```python
from build123d import *

# Parameters (mm, degrees)
SALIENTE_EXTRUIR1_DEPTH    = 3
SALIENTE_EXTRUIR2_DEPTH    = 3
NERVIO6_START              = -1.25
NERVIO6_DEPTH              = 2.5
NERVIO7_START              = -2
NERVIO7_DEPTH              = 4
CROQUIS3_R                 = 1.5875
CORTAR_EXTRUIR1_DEPTH      = 12
CORTAR_EXTRUIR2_DEPTH      = 10
CORTAR_EXTRUIR2_DEPTH_BACK = 12


# Read off the part's stored shape, not the designer's step: Nervio6, Nervio7
with BuildPart() as part:
    # Croquis1 → Saliente-Extruir1 (new body)
    with BuildSketch(Plane.XY):
        Polygon((-20, 5), (-20, -5), (20, -5), (20, 5), (0, 5), align=None)
        Polygon((-15, 30), (-20, 5), (0, 5), (0, 30), align=None)
        Polygon((0, 5), (20, 5), (15, 30), (0, 30), align=None)
    extrude(amount=SALIENTE_EXTRUIR1_DEPTH)

    # Croquis2 → Saliente-Extruir2 (add)
    with BuildSketch(Plane.XY.offset(3)):
        Polygon((-19.6, 7), (-20, 5), (20, 5), (19.6, 7), align=None)
    extrude(amount=SALIENTE_EXTRUIR2_DEPTH)

    # Nervio6 outline → Nervio6 (add)
    with BuildSketch(Plane(origin=(16, 0, 0), x_dir=(0, 0, -1), z_dir=(1, 0, 0)).offset(NERVIO6_START)):
        with BuildLine():
            Line((-3, 7), (-3, 18.5))
            ThreePointArc((-3, 18.5), (-3.776888017, 12.561362091), (-6, 7))
            Line((-6, 7), (-3, 7))
        make_face()
    nervio6 = extrude(amount=NERVIO6_DEPTH)

    # Simetría2: Nervio6 across plane
    add(nervio6.mirror(Plane(origin=(0, 0, 0), x_dir=(0, 0, 1), z_dir=(1, 0, 0))))

    # Nervio7 outline → Nervio7 (add)
    with BuildSketch(Plane(origin=(0, 0, 0), x_dir=(0, 0, -1), z_dir=(1, 0, 0)).offset(NERVIO7_START)):
        with BuildLine():
            Line((-3, 7), (-3, 11.670256173))
            ThreePointArc((-3, 11.670256173), (-3.927457039, 8.967347644), (-6, 7))
            Line((-6, 7), (-3, 7))
        make_face()
    extrude(amount=NERVIO7_DEPTH)

    # Croquis3 → Cortar-Extruir1 (cut)
    with BuildSketch(Plane.XY.offset(3)):
        with Locations((-12, 0)):
            Circle(CROQUIS3_R)
        with Locations((12, 0)):
            Circle(CROQUIS3_R)
    extrude(amount=-CORTAR_EXTRUIR1_DEPTH, mode=Mode.SUBTRACT)

    # Croquis4 → Cortar-Extruir2 (cut, two sides: drawn at the far end of the back side and taken through both)
    with BuildSketch(Plane.XY.offset(3).offset(-CORTAR_EXTRUIR2_DEPTH_BACK)):
        with BuildLine():
            Line((-12.5, 27), (12.5, 27))
            ThreePointArc((12.5, 27), (14.25, 25.25), (12.5, 23.5))
            Line((12.5, 23.5), (-12.5, 23.5))
            ThreePointArc((-12.5, 23.5), (-14.25, 25.25), (-12.5, 27))
        make_face()
        with BuildLine():
            Line((-12.5, 11.5), (12.5, 11.5))
            ThreePointArc((12.5, 11.5), (14.25, 13.25), (12.5, 15))
            Line((12.5, 15), (-12.5, 15))
            ThreePointArc((-12.5, 15), (-14.25, 13.25), (-12.5, 11.5))
        make_face()
    extrude(amount=CORTAR_EXTRUIR2_DEPTH + CORTAR_EXTRUIR2_DEPTH_BACK, mode=Mode.SUBTRACT)


solid = part.part
```
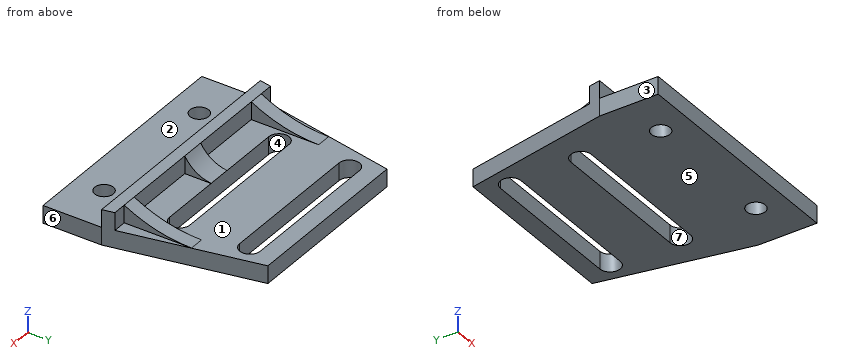
Check sheet for the modelled part. Datum: model origin and axes. Units: mm. Face numbers are marked on the shaded views. A direction names the side the tool comes from. Coordinates: 2 decimals unless noted, no trailing zeros. Loops run counter-clockwise (first coordinate to the right, second up) from the corner with the lowest first, then second, coordinate; pieces in that order, holes last.
1) Sectioned sample at B-B (y = 0). Record the boundary of the cut face in (x, z), and give its area (3 significant figures).
2) Access from +Z, -Z, +X, -X, +Y, -Y to the whole of each face (thin tool, end or side, straight path). Record for the marked faces 1, 2, 3 and 4.
3) Release check for a two-part mould opening along X. For the marked faces 5, 6 and 7 record: released by +X, released by -X, zero draft, split by the parting line, or undercut.
4) Sectioned sample at A-A (x = 0.5). Record the boundary of the cut face in (y, z).
5) Material ranges on probe 1 along Y at (x, z) = (-7, 2.2); probe 2 along Y at (x, z) = (12, 1.7); probe 3 along Y at (x, z) = (14, 1.2), recorded low to high.
6) Gauge pin test, flat ends, axial feed: pin 1 (3.5 mm diameter, centred on y = 10, z = 4, fed in from +X); pin 2 (2.5 mm diameter, centred on y = 9, z = 5, fed in from -X); pin 3 (1.5 mm diameter, centred on y = 12.5, z = 4, fed in from +X). Record the tip position at first contact, or that the pin passes through.
7) Sectioned sample at D-D (y = 25.25). Record the boundary of the cut face in (x, z).
8) Sectioned sample at C-C (z = 0.9). Count the separate pieces of the cut face and the enclosed holes in it, and give its area (3 significant figures).
Check sheet entries:
1. outline: (-20, 0) - (-13.59, 0) - (-13.59, 3) - (-20, 3) - close; (-10.41, 0) - (10.41, 0) - (10.41, 3) - (-10.41, 3) - close; (13.59, 0) - (20, 0) - (20, 3) - (13.59, 3) - close
1. area: 101 mm2
2. face 1: +Z, +Y
2. face 2: +Z, +X, -X, -Y
2. face 3: +Z, -Z, -X, +Y, -Y
2. face 4: +Z, -Z
3. face 5: zero draft
3. face 6: released by +X
3. face 7: undercut
4. outline: (-5, 0) - (11.5, 0) - (11.5, 3.02) arc R6 cw to (7, 6) - (5, 6) - (5, 3) - (-5, 3) - close; (15, 0) - (23.5, 0) - (23.5, 3) - (15, 3) - close; (27, 0) - (30, 0) - (30, 3) - (27, 3) - close
5. probe 1: y = -5 to 11.5, 15 to 23.5, 27 to 30
5. probe 2: y = -5 to -1.59, 1.59 to 11.5, 15 to 23.5, 27 to 30
5. probe 3: y = -5 to 12.35, 14.15 to 24.35, 26.15 to 30
6. pin 1: stops at x = 19.29
6. pin 2: stops at x = -17.25
6. pin 3: stops at x = 17.25
7. outline: (-15.95, 0) - (-14.25, 0) - (-14.25, 3) - (-15.95, 3) - close; (14.25, 0) - (15.95, 0) - (15.95, 3) - (14.25, 3) - close
8. separate pieces: 1
8. enclosed holes: 4
8. area: 1,060 mm2
